Print and shaded views of the part. All mm, measured from the part's lowest x, y and z. A direction names the side the tool comes from. Round coordinates to 2 decimals unless told otherwise and drop trailing zeros. Order: outer loops, then holes, each group sorted by start corner. A loop starts at its lowest first (then second) coordinate and runs counter-clockwise, first axis right, second up. Notation, with made-up numbers: (25, 13.25) - (69, 13.25) arc R29 ccw to (69, 50.25) - close; hole circle Ø4 at (3, -27.75). An arc over 180 degrees is marked (long way). Return JSON: item names as keys, results as strings. Group by question number.
Item 1: Drop flat-ended pins along their axis: pin 1 (2 mm diameter, centred on x = 24.6, y = 15, fed in from +Z); pin 2 (5.5 mm diameter, centred on x = 6.6, y = 15, fed in from +Z); pin 3 (10 mm diameter, centred on y = 40.5, z = 6, fed in from -X); pin 4 (2 mm diameter, centred on x = 30, z = 17.5, fed in from -Y). Give the stop position or say it passes through.
Item 2: Saw through at D-D on y = 10. List the corners of the cut face in (x, z).
Item 3: Saw through at A-A on x = 15.6. List the corners of the cut face in (y, z).
Item 4: Tool access for the marked faces 1 and 2: list every direction of +Z, -Z, +X, -X, +Y, -Y with a clear straight run to the whole face (end or side of a thin tool).
Item 5: Probe probe 1 along Z at (x, y) = (6.5, 45); probe 2 along X at (y, z) = (20.5, 15.5); probe 3 along X at (y, z) = (10.5, 4). List the from-to ranges inside material, lowest first.
Item 6: Saw through at B-B on y = 40. List the corners of the cut face in (x, z), and give its area (3 significant figures).
Item 7: Saw through at C-C on z = 40. List the corners of the cut face in (x, y), and give its area (3 significant figures).
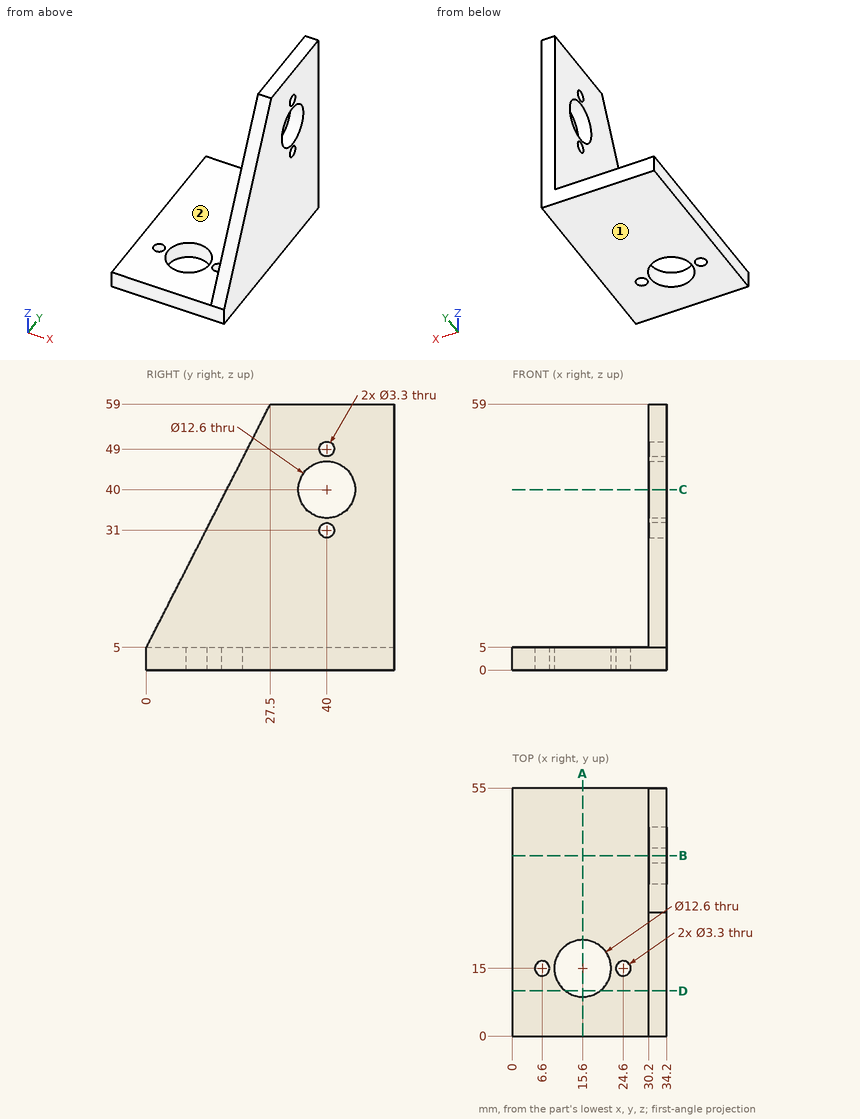
Filled in:
{
 "1": {"pin 1": "passes through", "pin 2": "stops at z = 5", "pin 3": "stops at x = 0", "pin 4": "stops at y = 5.87"},
 "2": {"outline": "(0, 0) - (11.77, 0) - (11.77, 5) - (0, 5) - close; (19.43, 0) - (34.2, 0) - (34.2, 24.64) - (30.2, 24.64) - (30.2, 5) - (19.43, 5) - close"},
 "3": {"outline": "(0, 0) - (8.7, 0) - (8.7, 5) - (0, 5) - close; (21.3, 0) - (55, 0) - (55, 5) - (21.3, 5) - close"},
 "4": {"face 1": "-Z, +X, -X, +Y, -Y", "face 2": "+Z, -X, +Y, -Y"},
 "5": {"probe 1": "z = 0 to 5", "probe 2": "x = 30.2 to 34.2", "probe 3": "x = 0 to 11.19, 20.01 to 34.2"},
 "6": {"outline": "(0, 0) - (34.2, 0) - (34.2, 29.35) - (30.2, 29.35) - (30.2, 5) - (0, 5) - close; (30.2, 32.65) - (34.2, 32.65) - (34.2, 33.7) - (30.2, 33.7) - close; (30.2, 46.3) - (34.2, 46.3) - (34.2, 47.35) - (30.2, 47.35) - close; (30.2, 50.65) - (34.2, 50.65) - (34.2, 59) - (30.2, 59) - close", "area": "310 mm^2"},
 "7": {"outline": "(30.2, 17.82) - (34.2, 17.82) - (34.2, 33.7) - (30.2, 33.7) - close; (30.2, 46.3) - (34.2, 46.3) - (34.2, 55) - (30.2, 55) - close", "area": "98.3 mm^2"}
}
